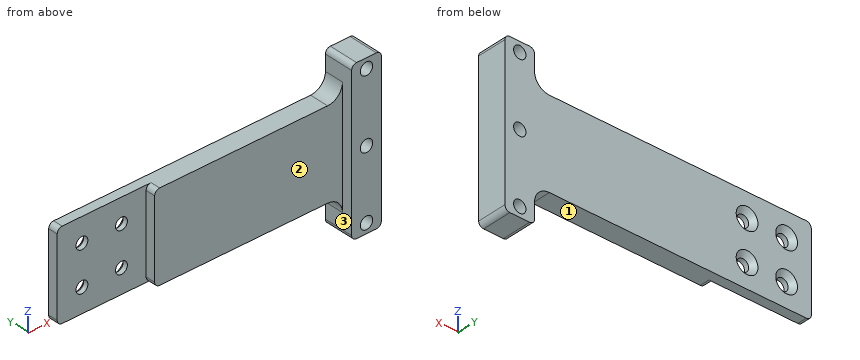
from build123d import *

# Parameters (mm, degrees)
BOSS_EXTRUDE1_DEPTH                                 = 3.9
BOSS_EXTRUDE2_DEPTH                                 = 2.1
CSK_FOR_M2_COUNTERSUNK_FLAT_HEAD_SCREW1_D           = 2.4
CSK_FOR_M2_COUNTERSUNK_FLAT_HEAD_SCREW1_CSINK_D     = 4.4
CSK_FOR_M2_COUNTERSUNK_FLAT_HEAD_SCREW1_CSINK_ANGLE = 90
LPATTERN1_COUNT                                     = 2
LPATTERN1_PITCH                                     = 8
LPATTERN1_COUNT_DIR2                                = 2
LPATTERN1_PITCH_DIR2                                = 8
SKETCH7_W                                           = 8
SKETCH7_H                                           = 6
CUT_EXTRUDE1_DEPTH                                  = 36.397740041
SKETCH10_W                                          = 18
SKETCH10_H                                          = 18
CUT_EXTRUDE2_DEPTH                                  = 1.95
SKETCH14_W                                          = 8
SKETCH14_H                                          = 1
CUT_EXTRUDE3_DEPTH                                  = 36.11983058
M3_TAPPED_HOLE1_D                                   = 2.5
M3_TAPPED_HOLE1_DEPTH                               = 6.748924226
M3_TAPPED_HOLE1_TIP                                 = 0.751075774
SKETCH15_W                                          = 56
SKETCH15_H                                          = 3.05
CUT_EXTRUDE4_DEPTH                                  = 36.397740041
FILLET5_R                                           = 1
FILLET7_R                                           = 3


with BuildPart() as part:
    # Sketch1 → Boss-Extrude1 (new body)
    with BuildSketch(Plane(origin=(0, 0, 0), x_dir=(1, 0, 0), z_dir=(0, 1, 0))):
        Polygon((22, 11.9), (25, 11.9), (25, 16), (28, 16), (31, 16), (31, -16), (28, -16), (25, -16), (25, -11.9), (22, -11.9), (-31, -11.9), (-31, 11.9), align=None)
    extrude(amount=BOSS_EXTRUDE1_DEPTH)

    # Sketch6 → Boss-Extrude2 (add)
    with BuildSketch(Plane.XZ):
        Polygon((25, 11.9), (25, 16), (28, 16), (31, 16), (31, -16), (28, -16), (25, -16), (25, -11.9), align=None)
    extrude(amount=BOSS_EXTRUDE2_DEPTH)

    # CSK for M2 Countersunk Flat Head Screw1 (through all)
    with Locations(Plane(origin=(0, 3.9, 0), x_dir=(1, 0, 0), z_dir=(0, 1, 0))):
        with Locations((-18, 4)):
            csk_for_m2_countersunk_flat_head_screw1 = CounterSinkHole(CSK_FOR_M2_COUNTERSUNK_FLAT_HEAD_SCREW1_D / 2, CSK_FOR_M2_COUNTERSUNK_FLAT_HEAD_SCREW1_CSINK_D / 2, counter_sink_angle=CSK_FOR_M2_COUNTERSUNK_FLAT_HEAD_SCREW1_CSINK_ANGLE)

    # LPattern1: CSK for M2 Countersunk Flat Head Screw1 2 × 2
    with Locations(*[(-i * LPATTERN1_PITCH, 0, j * LPATTERN1_PITCH_DIR2) for i in range(LPATTERN1_COUNT) for j in range(LPATTERN1_COUNT_DIR2) if (i, j) != (0, 0)]):
        add(csk_for_m2_countersunk_flat_head_screw1, mode=Mode.SUBTRACT)

    # Sketch7 → Cut-Extrude1 (cut, through all)
    with BuildSketch(Plane(origin=(0, 3.9, 0), x_dir=(1, 0, 0), z_dir=(0, 1, 0))):
        with Locations((-27, 12)):
            Rectangle(SKETCH7_W, SKETCH7_H)
        with Locations((-27, -12)):
            Rectangle(SKETCH7_W, SKETCH7_H)
    extrude(amount=-CUT_EXTRUDE1_DEPTH, mode=Mode.SUBTRACT)

    # Sketch10 → Cut-Extrude2 (cut)
    with BuildSketch(Plane.XZ):
        with Locations((-22, 0)):
            Rectangle(SKETCH10_W, SKETCH10_H)
    extrude(amount=-CUT_EXTRUDE2_DEPTH, mode=Mode.SUBTRACT)

    # Sketch14 → Cut-Extrude3 (cut, through all)
    with BuildSketch(Plane.XZ.offset(-1.95)):
        with Locations((-27, -9.45)):
            Rectangle(SKETCH14_W, SKETCH14_H)
        with Locations((-27, 9.45)):
            Rectangle(SKETCH14_W, SKETCH14_H)
    extrude(amount=-CUT_EXTRUDE3_DEPTH, mode=Mode.SUBTRACT)

    # M3 Tapped Hole1
    with Locations(Plane(origin=(0, 3.9, 0), x_dir=(1, 0, 0), z_dir=(0, 1, 0))):
        with Locations((28, 14), (28, -14), (28, 0)):
            Hole(M3_TAPPED_HOLE1_D / 2, depth=M3_TAPPED_HOLE1_DEPTH)
            with Locations((0, 0, -(M3_TAPPED_HOLE1_DEPTH + M3_TAPPED_HOLE1_TIP / 2))):  # 118° drill point
                Cone(0, M3_TAPPED_HOLE1_D / 2, M3_TAPPED_HOLE1_TIP, mode=Mode.SUBTRACT)

    # Sketch15 → Cut-Extrude4 (cut, through all)
    with BuildSketch(Plane(origin=(0, 3.9, 0), x_dir=(1, 0, 0), z_dir=(0, 1, 0))):
        with Locations((-3, 10.375)):
            Rectangle(SKETCH15_W, SKETCH15_H)
        with Locations((-3, -10.375)):
            Rectangle(SKETCH15_W, SKETCH15_H)
    extrude(amount=-CUT_EXTRUDE4_DEPTH, mode=Mode.SUBTRACT)

    # Fillet5
    fillet5_edges = [part.edges().sort_by_distance(p)[0] for p in [
        (25, 0.9, -16),
        (31, 0.9, -16),
        (31, 0.9, 16),
        (25, 0.9, 16),
        (-13, 0.975, 8.85),
        (-13, 0.975, -8.85),
        (-31, 2.925, -8.85),
        (-31, 2.925, 8.85),
    ]]
    fillet(fillet5_edges, radius=FILLET5_R)

    # Fillet7
    fillet7_edges = [part.edges().sort_by_distance(p)[0] for p in [
        (25, 1.95, -8.85),
        (25, 1.95, 8.85),
    ]]
    fillet(fillet7_edges, radius=FILLET7_R)


solid = part.part
Input: part model. Units: mm. Frame: model coordinates. Face numbers are marked on the shaded views. A direction names the side the tool comes from. Coordinates: 2 decimals unless noted, no trailing zeros. Write each loop counter-clockwise with the first axis right and the second up, starting at its lowest first coordinate (ties: lowest second). Pieces come first, ordered by that corner, then holes. Notation, with made-up numbers: M 74,-38.75 L 92,-38.75 A32 ccw 92,-11.75 Z; hole C 63,46 d7. An arc over 180 degrees is marked long. Answer as a JSON object with one key per item and string values. Group by question number.
(1) Section B-B on z = 0. Output: boundary loops of the cut face in (x, y), plus the area to 3 significant figures.
(2) Section A-A on x = -18. Output: boundary loops of the cut face in (y, z), plus the area to 3 significant figures.
(3) Section C-C on z = -4. Output: boundary loops of the cut face in (x, y).
(4) Section D-D on y = -1.4. Output: boundary loops of the cut face in (x, z), plus the area to 3 significant figures.
(5) Ray query, line 1 along Z through (x, y) = (-18, 2.3); line 2 along X through (y, z) = (0.05, -14); line 3 along X through (y, z) = (0.3, 3.5). Return the intervals inside material, ascending. Write a range as [from, to].
(6) Contact query for flat-ended pins moving along their axis: P1, Ø4, axis at x = -18, z = -4, coming from the -Y side; P2, Ø3, axis at x = 3.5, y = 2, coming from the -Z side; P3, Ø3, axis at x = -26, z = -4, coming from the +Y side. Output: stop coordinate, or through.
(7) Set-up query: the marked faces 1, 2 and 3. Return all of +Z, -Z, +X, -X, +Y, -Y with unobstructed straight access to the full face (end or side cutting, diameter ignored); none if empty.
Result set:
{
 "1": {"outline": "M -31,1.95 L -13,1.95 L -13,0 L 25,0 L 25,-2.1 L 26.75,-2.1 L 26.75,3.9 L -31,3.9 Z; M 29.25,-2.1 L 31,-2.1 L 31,3.9 L 29.25,3.9 Z", "area": "204 mm2"},
 "2": {"outline": "M 1.95,-8.85 L 3.9,-8.85 L 3.9,-6.2 L 2.9,-5.2 L 1.95,-5.2 Z; M 1.95,-2.8 L 2.9,-2.8 L 3.9,-1.8 L 3.9,1.8 L 2.9,2.8 L 1.95,2.8 Z; M 1.95,5.2 L 2.9,5.2 L 3.9,6.2 L 3.9,8.85 L 1.95,8.85 Z", "area": "23.2 mm2"},
 "3": {"outline": "M -31,1.95 L -27.2,1.95 L -27.2,2.9 L -28.2,3.9 L -31,3.9 Z; M -24.8,1.95 L -19.2,1.95 L -19.2,2.9 L -20.2,3.9 L -23.8,3.9 L -24.8,2.9 Z; M -16.8,1.95 L -13,1.95 L -13,0 L 25,0 L 25,-2.1 L 31,-2.1 L 31,3.9 L -15.8,3.9 L -16.8,2.9 Z"},
 "4": {"outline": "M 25,-15 A1 ccw 26,-16 L 30,-16 A1 ccw 31,-15 L 31,15 A1 ccw 30,16 L 26,16 A1 ccw 25,15 Z; hole C 28,-14 d2.5; hole C 28,0 d2.5; hole C 28,14 d2.5", "area": "176 mm2"},
 "5": {"line 1": "z = [-8.85, -5.2], [-2.8, 2.8], [5.2, 8.85]", "line 2": "x = [25, 26.75], [29.25, 31]", "line 3": "x = [-13, 31]"},
 "6": {"P1": "stops at y = 1.95", "P2": "stops at z = -8.85", "P3": "stops at y = 3.2"},
 "7": {"face 1": "-Z, -X, +Y, -Y", "face 2": "+Z, -Z, -X, -Y", "face 3": "-X, -Y"}
}
